Work out the finished part from the listing and answer in its coordinate system (mm). A direction names the side the tool comes from. Round coordinates to 2 decimals unless told otherwise and drop trailing zeros. Order: outer loops, then holes, each group sorted by start corner. A loop starts at its lowest first (then second) coordinate and runs counter-clockwise, first axis right, second up. Notation, with made-up numbers: M 29.5,66.5 L 86.5,66.5 A4 ccw 86.5,72.5 Z; hole C 3.5,51.5 d2. An arc over 180 degrees is marked long. Return JSON: item names as keys, results as strings.
from build123d import *

# Parameters (mm, degrees)
SKETCH1_W                       = 100
SKETCH1_H                       = 150
BOSS_EXTRUDE1_DEPTH             = 25
TAP_DRILL_FOR_M5X0_8_TAP1_D     = 4.2
TAP_DRILL_FOR_M5X0_8_TAP1_DEPTH = 20
TAP_DRILL_FOR_M5X0_8_TAP1_TIP   = 1.2618073
CUT_EXTRUDE1_DEPTH              = 45
SKETCH6_W                       = 12.7
SKETCH6_H                       = 13
CUT_EXTRUDE2_DEPTH              = 2.54
FILLET1_R                       = 6
FILLET3_R                       = 2.5
CHAMFER1_SIZE                   = 1


with BuildPart() as part:
    # Sketch1 → Boss-Extrude1 (new, symmetric)
    with BuildSketch(Plane(origin=(0, 0, 0), x_dir=(1, 0, 0), z_dir=(0, 1, 0))):
        Rectangle(SKETCH1_W, SKETCH1_H)
    extrude(amount=BOSS_EXTRUDE1_DEPTH, both=True)

    # Tap Drill for M5x0.8 Tap1
    with Locations(Plane(origin=(-42.5, 25, -67.5), x_dir=(0, 0, 1), z_dir=(0, 1, 0))):
        with Locations((0, 0), (0, 85), (135, 85), (135, 0)):
            Hole(TAP_DRILL_FOR_M5X0_8_TAP1_D / 2, depth=TAP_DRILL_FOR_M5X0_8_TAP1_DEPTH)
            with Locations((0, 0, -(TAP_DRILL_FOR_M5X0_8_TAP1_DEPTH + TAP_DRILL_FOR_M5X0_8_TAP1_TIP / 2))):  # 118° drill point
                Cone(0, TAP_DRILL_FOR_M5X0_8_TAP1_D / 2, TAP_DRILL_FOR_M5X0_8_TAP1_TIP, mode=Mode.SUBTRACT)

    # Sketch5 → Cut-Extrude1 (cut)
    with BuildSketch(Plane(origin=(0, 25, 0), x_dir=(1, 0, 0), z_dir=(0, 1, 0))):
        with BuildLine():
            Line((-45, 60.85470091), (-45, -60.85470091))
            ThreePointArc((-45, -60.85470091), (-37.479541854, -62.479541854), (-35.85470091, -70))
            Line((-35.85470091, -70), (-11.35, -70))
            Line((-11.35, -70), (-11.35, -62))
            Line((-11.35, -62), (11.35, -62))
            Line((11.35, -62), (11.35, -70))
            Line((11.35, -70), (35.85470091, -70))
            ThreePointArc((35.85470091, -70), (37.479541854, -62.479541854), (45, -60.85470091))
            Line((45, -60.85470091), (45, 60.85470091))
            ThreePointArc((45, 60.85470091), (37.479541854, 62.479541854), (35.85470091, 70))
            Line((35.85470091, 70), (-35.85470091, 70))
            ThreePointArc((-35.85470091, 70), (-37.479541854, 62.479541854), (-45, 60.85470091))
        make_face()
    extrude(amount=-CUT_EXTRUDE1_DEPTH, mode=Mode.SUBTRACT)

    # Sketch6 → Cut-Extrude2 (cut)
    with BuildSketch(Plane(origin=(0, 25, 0), x_dir=(1, 0, 0), z_dir=(0, 1, 0))):
        with Locations((0, -68.5)):
            Rectangle(SKETCH6_W, SKETCH6_H)
    extrude(amount=-CUT_EXTRUDE2_DEPTH, mode=Mode.SUBTRACT)

    # Fillet1
    fillet1_edges = [part.edges().sort_by_distance(p)[0] for p in [
        (-45, 2.5, 60.85470091),
        (-35.85470091, 2.5, 70),
        (-11.35, 2.5, 70),
        (11.35, 2.5, 70),
        (35.85470091, 2.5, 70),
        (45, 2.5, 60.85470091),
        (45, 2.5, -60.85470091),
        (35.85470091, 2.5, -70),
        (-35.85470091, 2.5, -70),
        (-45, 2.5, -60.85470091),
        (50, 0, 75),
        (-50, 0, 75),
        (-50, 0, -75),
        (50, 0, -75),
    ]]
    fillet(fillet1_edges, radius=FILLET1_R)

    # Fillet3
    fillet3_edges = [part.edges().sort_by_distance(p)[0] for p in [
        (11.35, 2.5, 62),
        (-11.35, 2.5, 62),
    ]]
    fillet(fillet3_edges, radius=FILLET3_R)

    # Chamfer1
    chamfer1_edges = [part.edges().sort_by_distance(p)[0] for p in [
        (25.175, 25, 75),
        (0, 25, -75),
        (50, 25, 0),
        (-50, 25, 0),
        (-25.175, 25, 75),
        (48.242640687, 25, 73.242640687),
        (-48.242640687, 25, 73.242640687),
        (-48.242640687, 25, -73.242640687),
        (48.242640687, 25, -73.242640687),
    ]]
    chamfer(chamfer1_edges, length=CHAMFER1_SIZE)


solid = part.part
Item 1: Each of these flat-tipped pins is pushed along its axis until it touches: pin 1 (6 mm diameter, centred on x = 17.5, z = 3, fed in from +Y); pin 2 (1.3 mm diameter, centred on y = 24, z = 71, fed in from -X). Where does it stop, or does it pass through?
Output:
{"pin 1": "stops at y = -20", "pin 2": "stops at x = -49.85"}
Item 2: Find section D-D (x = 0). Determine the outline of the cut face in (y, z), plus the area to 3 significant figures.
Output:
{"outline": "M -25,-75 L 24,-75 L 25,-74 L 25,-70 L -20,-70 L -20,62 L 22.46,62 L 22.46,75 L -25,75 Z", "area": "1,530 mm^2"}
Item 3: Find section A-A (z = 41.5). Determine the outline of the cut face in (x, y), plus the area to 3 significant figures.
Output:
{"outline": "M -50,-25 L 50,-25 L 50,24 L 49,25 L 45,25 L 45,-20 L -45,-20 L -45,25 L -49,25 L -50,24 Z", "area": "949 mm^2"}
Item 4: Consider line 1 along Z through (x, y) = (-0.5, -19); line 2 along Z through (x, y) = (-42.5, 18.5); line 3 along Z through (x, y) = (44, 14). Determine where each line is inside the solid, lowest interval first. Write a range as [from, to].
Output:
{"line 1": "z = [-75, -70], [62, 75]", "line 2": "z = [-75, -69.6], [-65.4, -59.75], [59.75, 65.4], [69.6, 75]", "line 3": "z = [-75, -68.97], [-66.03, -58.19], [58.19, 66.03], [68.97, 75]"}
Item 5: Find section C-C (y = 6.5). State how many separate pieces and enclosed holes the cut face has, plus the area to 3 significant figures.
Output:
{"separate pieces": "1", "enclosed holes": "5", "area": "2,880 mm^2"}
Item 6: The mould has two halves that part along Z. Classify faces 3 (the cylindrical face through (-48.289, -0.843, -73.196)), 4 (the flat face through (0, 22.46, 68)), 5 (the cylindrical face through (37.44, 2.82, 62.52)): pulls with the +Z half, pulls with the -Z half, needs draft (parallel to the pull), parting line crosses it, or undercut.
Output:
{"face 3": "pulls with the -Z half", "face 4": "needs draft", "face 5": "undercut"}
Item 7: Find section B-B (x = -21.5). Determine the outline of the cut face in (y, z), plus the area to 3 significant figures.
Output:
{"outline": "M -25,-75 L 24,-75 L 25,-74 L 25,-70 L -20,-70 L -20,70 L 25,70 L 25,74 L 24,75 L -25,75 Z", "area": "1,200 mm^2"}
Item 8: Which of the six approach directions +Z, -Z, +X, -X, +Y, -Y give full straight-line access (tool end or side, diameter ignored) to faces 1 (the cylindrical face through (-48.289, -0.157, 73.196)), 2 (the cylindrical face through (40.637, 14.86, 66.531))?
Output:
{"face 1": "+Z, -X, +Y, -Y", "face 2": "+Y"}
